Could you check a few things on this model? Use its own coordinates, in mm. A direction names the side the tool comes from. Coordinates: 2 decimals unless noted, no trailing zeros. Order: outer loops, then holes, each group sorted by start corner. A loop starts at its lowest first (then second) coordinate and runs counter-clockwise, first axis right, second up. Notation, with made-up numbers: (85, 24) - (140, 24) arc R27 ccw to (140, 53) - close; hole circle Ø9 at (3.25, 0.25). An arc over 180 degrees is marked (long way). One line per item, written item: value.
from build123d import *

# Parameters (mm, degrees)
SKETCH1_W           = 50
SKETCH1_H           = 22.5
SKETCH1_R           = 3
BOSS_EXTRUDE1_DEPTH = 3
SKETCH3_W           = 50
SKETCH3_H           = 22.5
SKETCH3_R           = 3
BOSS_EXTRUDE2_DEPTH = 3


with BuildPart() as part:
    # Sketch1 → Boss-Extrude1 (new body)
    with BuildSketch(Plane.XY):
        with Locations((-17.806163097, -13.303318659)):
            Rectangle(SKETCH1_W, SKETCH1_H)
        with Locations((-2.806163097, -17.053318659)):
            Circle(SKETCH1_R, mode=Mode.SUBTRACT)
        with Locations((-32.806163097, -17.053318659)):
            Circle(SKETCH1_R, mode=Mode.SUBTRACT)
    extrude(amount=BOSS_EXTRUDE1_DEPTH)

    # Sketch3 → Boss-Extrude2 (add)
    with BuildSketch(Plane(origin=(0, -2.053318659, 0), x_dir=(1, 0, 0), z_dir=(0, 1, 0))):
        with Locations((-17.806163097, -11.25)):
            Rectangle(SKETCH3_W, SKETCH3_H)
        with Locations((-2.806163097, -15)):
            Circle(SKETCH3_R, mode=Mode.SUBTRACT)
        with Locations((-32.806163097, -15)):
            Circle(SKETCH3_R, mode=Mode.SUBTRACT)
    extrude(amount=BOSS_EXTRUDE2_DEPTH)


solid = part.part
Item 1: I want a section at B-B on y = -18. Please give me the cut outline in (x, z), then the cut area to 3 significant figures.
Conclusion:
outline: (-42.81, 0) - (-35.65, 0) - (-35.65, 3) - (-42.81, 3) - close; (-29.96, 0) - (-5.65, 0) - (-5.65, 3) - (-29.96, 3) - close; (0.04, 0) - (7.19, 0) - (7.19, 3) - (0.04, 3) - close
area: 116 mm²
Item 2: I'm going to push flat-ended pins straight in: pin 1 Ø7 at (x, y) = (-2.81, -17.05) entering from +Z; pin 2 Ø2 at (y, z) = (-13.5, 4.5) entering from +X; pin 3 Ø8 at (x, z) = (-2.81, 15) entering from -Y. Where does each tip first touch, or does it pass through?
Conclusion:
pin 1: z = 3
pin 2: through
pin 3: y = -2.05
Item 3: I want a section at A-A on z = 15. Please give me the cut outline in (x, y).
Conclusion:
outline: (-42.81, -2.05) - (-35.81, -2.05) - (-35.81, 0.95) - (-42.81, 0.95) - close; (-29.81, -2.05) - (-5.81, -2.05) - (-5.81, 0.95) - (-29.81, 0.95) - close; (0.19, -2.05) - (7.19, -2.05) - (7.19, 0.95) - (0.19, 0.95) - close
Item 4: For faces 5 (the face through (-18, -13, 3)), 6 (the face through (-18, -24.553, 1)), which set-ups out of +Z, -Z, +X, -X, +Y, -Y let a thin tool reach every point of the face, with its end or its side?
Conclusion:
face 5: +Z, +X, -X, -Y
face 6: +Z, -Z, +X, -X, -Y
Item 5: I want a section at C-C on x = -26.5. Please give me the cut outline in (y, z), then the cut area to 3 significant figures.
Conclusion:
outline: (-24.55, 0) - (0.95, 0) - (0.95, 22.5) - (-2.05, 22.5) - (-2.05, 3) - (-24.55, 3) - close
area: 135 mm²
Item 6: If I drill on probe 1 along X at (y, z) = (-0.65, 15); probe 2 along Z at (x, y) = (-39, -7.5); probe 3 along Y at (x, z) = (-33.5, 18.5), over which ranges is the centre line in solid material (lowest first)?
Conclusion:
probe 1: -42.81 to -35.81, -29.81 to -5.81, 0.19 to 7.19
probe 2: 0 to 3
probe 3: -2.05 to 0.95
Item 7: I want a section at D-D on y = -22.75. Please give me the cut outline in (x, z).
Conclusion:
outline: (-42.81, 0) - (7.19, 0) - (7.19, 3) - (-42.81, 3) - close
Item 8: Thinking about a two-plate mould opening in Y: for faces 1 (the face through (-31.193, -14.524, 1.479)), 2 (the face through (-1.193, -14.524, 1.479)), 3 (the face through (7.194, -7, 2)), 4 (the face through (-18, -2.053, 13)), which applies, pulls with the +Y half, pulls with the -Y half, needs draft (parallel to the pull), parting line crosses it, or undercut?
Conclusion:
face 1: undercut
face 2: undercut
face 3: needs draft
face 4: pulls with the -Y half
